from build123d import *

# Parameters (mm, degrees)
EXTRUDE_1_DEPTH = 3


with BuildPart() as part:
    # 草图1 → 凸台-拉伸1 (new body)
    with BuildSketch(Plane(origin=(0, 0, 0), x_dir=(-1, 0, 0), z_dir=(0, 0, 1))):
        with BuildLine():
            Line((-132.77617551, 2.029328632), (-134.77617551, 4.029328632))
            Line((-134.77617551, 4.029328632), (-144.77617551, 4.029328632))
            Line((-144.77617551, 4.029328632), (-144.77617551, 0.948486637))
            Line((-144.77617551, 0.948486637), (-156.77617551, 0.948486637))
            Line((-156.77617551, 0.948486637), (-156.77617551, 4.029328632))
            Line((-156.77617551, 4.029328632), (-181.77617551, 4.029328632))
            Line((-181.77617551, 4.029328632), (-181.77617551, 0.948486637))
            Line((-181.77617551, 0.948486637), (-195.77617551, 0.948486637))
            Line((-195.77617551, 0.948486637), (-195.77617551, 5.029328632))
            Line((-195.77617551, 5.029328632), (-207.77617551, 5.029328632))
            Line((-207.77617551, 5.029328632), (-207.77617551, 0.948486637))
            Line((-207.77617551, 0.948486637), (-221.77617551, 0.948486637))
            Line((-221.77617551, 0.948486637), (-221.77617551, 4.029328632))
            Line((-221.77617551, 4.029328632), (-246.77617551, 4.029328632))
            Line((-246.77617551, 4.029328632), (-246.77617551, 0.948486637))
            Line((-246.77617551, 0.948486637), (-258.77617551, 0.948486637))
            Line((-258.77617551, 0.948486637), (-258.77617551, 4.029328632))
            Line((-258.77617551, 4.029328632), (-268.77617551, 4.029328632))
            Line((-268.77617551, 4.029328632), (-270.77617551, 2.029328632))
            Line((-270.77617551, 2.029328632), (-270.77617551, -41.970671368))
            ThreePointArc((-270.77617551, -41.970671368), (-272.240641604, -45.506205274), (-275.77617551, -46.970671368))
            Line((-275.77617551, -46.970671368), (-296.77617551, -46.970671368))
            ThreePointArc((-296.77617551, -46.970671368), (-298.190389072, -47.556457806), (-298.77617551, -48.970671368))
            Line((-298.77617551, -48.970671368), (-298.77617551, -61.470671368))
            ThreePointArc((-298.77617551, -61.470671368), (-292.125960742, -70.210089556), (-282.77617551, -75.970671368))
            Line((-282.77617551, -75.970671368), (-274.77617551, -75.970671368))
            Line((-274.77617551, -75.970671368), (-272.77617551, -73.970671368))
            Line((-272.77617551, -73.970671368), (-272.77617551, -66.665321612))
            ThreePointArc((-272.77617551, -66.665321612), (-271.897495853, -64.544001269), (-269.77617551, -63.665321612))
            Line((-269.77617551, -63.665321612), (-266.77617551, -63.665321612))
            Line((-266.77617551, -63.665321612), (-266.77617551, -53.665321612))
            Line((-266.77617551, -53.665321612), (-262.77617551, -53.665321612))
            Line((-262.77617551, -53.665321612), (-262.77617551, -63.665321612))
            Line((-262.77617551, -63.665321612), (-248.77617551, -63.665321612))
            Line((-248.77617551, -63.665321612), (-242.77617551, -57.665321612))
            Line((-242.77617551, -57.665321612), (-242.77617551, -19.470671368))
            Line((-242.77617551, -19.470671368), (-235.77617551, -19.470671368))
            Line((-235.77617551, -19.470671368), (-235.77617551, -25.415321612))
            Line((-235.77617551, -25.415321612), (-231.17617551, -25.415321612))
            Line((-231.17617551, -25.415321612), (-231.17617551, -23.370671368))
            Line((-231.17617551, -23.370671368), (-232.22617551, -23.370671368))
            ThreePointArc((-232.22617551, -23.370671368), (-232.438307544, -23.282803402), (-232.52617551, -23.070671368))
            Line((-232.52617551, -23.070671368), (-232.52617551, -21.170671368))
            ThreePointArc((-232.52617551, -21.170671368), (-232.438307544, -20.958539334), (-232.22617551, -20.870671368))
            Line((-232.22617551, -20.870671368), (-231.12617551, -20.870671368))
            Line((-231.12617551, -20.870671368), (-231.12617551, -20.670671368))
            ThreePointArc((-231.12617551, -20.670671368), (-231.038307544, -20.458539334), (-230.82617551, -20.370671368))
            Line((-230.82617551, -20.370671368), (-228.72617551, -20.370671368))
            ThreePointArc((-228.72617551, -20.370671368), (-228.514043475, -20.458539334), (-228.42617551, -20.670671368))
            Line((-228.42617551, -20.670671368), (-228.42617551, -20.870671368))
            Line((-228.42617551, -20.870671368), (-227.32617551, -20.870671368))
            ThreePointArc((-227.32617551, -20.870671368), (-227.114043475, -20.958539334), (-227.02617551, -21.170671368))
            Line((-227.02617551, -21.170671368), (-227.02617551, -23.070671368))
            ThreePointArc((-227.02617551, -23.070671368), (-227.114043475, -23.282803402), (-227.32617551, -23.370671368))
            Line((-227.32617551, -23.370671368), (-228.37617551, -23.370671368))
            Line((-228.37617551, -23.370671368), (-228.37617551, -25.415321612))
            Line((-228.37617551, -25.415321612), (-224.77617551, -25.415321612))
            Line((-224.77617551, -25.415321612), (-224.77617551, -30.915321612))
            Line((-224.77617551, -30.915321612), (-214.77617551, -30.915321612))
            Line((-214.77617551, -30.915321612), (-214.77617551, -25.415321612))
            Line((-214.77617551, -25.415321612), (-203.17617551, -25.415321612))
            Line((-203.17617551, -25.415321612), (-203.17617551, -23.370671368))
            Line((-203.17617551, -23.370671368), (-204.22617551, -23.370671368))
            ThreePointArc((-204.22617551, -23.370671368), (-204.438307544, -23.282803402), (-204.52617551, -23.070671368))
            Line((-204.52617551, -23.070671368), (-204.52617551, -21.170671368))
            ThreePointArc((-204.52617551, -21.170671368), (-204.438307544, -20.958539334), (-204.22617551, -20.870671368))
            Line((-204.22617551, -20.870671368), (-203.12617551, -20.870671368))
            Line((-203.12617551, -20.870671368), (-203.12617551, -20.670671368))
            ThreePointArc((-203.12617551, -20.670671368), (-203.038307544, -20.458539334), (-202.82617551, -20.370671368))
            Line((-202.82617551, -20.370671368), (-200.72617551, -20.370671368))
            ThreePointArc((-200.72617551, -20.370671368), (-200.514043475, -20.458539334), (-200.42617551, -20.670671368))
            Line((-200.42617551, -20.670671368), (-200.42617551, -20.870671368))
            Line((-200.42617551, -20.870671368), (-199.32617551, -20.870671368))
            ThreePointArc((-199.32617551, -20.870671368), (-199.114043475, -20.958539334), (-199.02617551, -21.170671368))
            Line((-199.02617551, -21.170671368), (-199.02617551, -23.070671368))
            ThreePointArc((-199.02617551, -23.070671368), (-199.114043475, -23.282803402), (-199.32617551, -23.370671368))
            Line((-199.32617551, -23.370671368), (-200.37617551, -23.370671368))
            Line((-200.37617551, -23.370671368), (-200.37617551, -25.415321612))
            Line((-200.37617551, -25.415321612), (-188.77617551, -25.415321612))
            Line((-188.77617551, -25.415321612), (-188.77617551, -30.915321612))
            Line((-188.77617551, -30.915321612), (-178.77617551, -30.915321612))
            Line((-178.77617551, -30.915321612), (-178.77617551, -25.415321612))
            Line((-178.77617551, -25.415321612), (-175.17617551, -25.415321612))
            Line((-175.17617551, -25.415321612), (-175.17617551, -23.370671368))
            Line((-175.17617551, -23.370671368), (-176.22617551, -23.370671368))
            ThreePointArc((-176.22617551, -23.370671368), (-176.438307544, -23.282803402), (-176.52617551, -23.070671368))
            Line((-176.52617551, -23.070671368), (-176.52617551, -21.170671368))
            ThreePointArc((-176.52617551, -21.170671368), (-176.438307544, -20.958539334), (-176.22617551, -20.870671368))
            Line((-176.22617551, -20.870671368), (-175.12617551, -20.870671368))
            Line((-175.12617551, -20.870671368), (-175.12617551, -20.670671368))
            ThreePointArc((-175.12617551, -20.670671368), (-175.038307544, -20.458539334), (-174.82617551, -20.370671368))
            Line((-174.82617551, -20.370671368), (-172.72617551, -20.370671368))
            ThreePointArc((-172.72617551, -20.370671368), (-172.514043475, -20.458539334), (-172.42617551, -20.670671368))
            Line((-172.42617551, -20.670671368), (-172.42617551, -20.870671368))
            Line((-172.42617551, -20.870671368), (-171.32617551, -20.870671368))
            ThreePointArc((-171.32617551, -20.870671368), (-171.114043475, -20.958539334), (-171.02617551, -21.170671368))
            Line((-171.02617551, -21.170671368), (-171.02617551, -23.070671368))
            ThreePointArc((-171.02617551, -23.070671368), (-171.114043475, -23.282803402), (-171.32617551, -23.370671368))
            Line((-171.32617551, -23.370671368), (-172.37617551, -23.370671368))
            Line((-172.37617551, -23.370671368), (-172.37617551, -25.415321612))
            Line((-172.37617551, -25.415321612), (-167.77617551, -25.415321612))
            Line((-167.77617551, -25.415321612), (-167.77617551, -19.470671368))
            Line((-167.77617551, -19.470671368), (-160.77617551, -19.470671368))
            Line((-160.77617551, -19.470671368), (-160.77617551, -57.665321612))
            Line((-160.77617551, -57.665321612), (-154.77617551, -63.665321612))
            Line((-154.77617551, -63.665321612), (-140.77617551, -63.665321612))
            Line((-140.77617551, -63.665321612), (-140.77617551, -53.665321612))
            Line((-140.77617551, -53.665321612), (-136.77617551, -53.665321612))
            Line((-136.77617551, -53.665321612), (-136.77617551, -63.665321612))
            Line((-136.77617551, -63.665321612), (-133.77617551, -63.665321612))
            ThreePointArc((-133.77617551, -63.665321612), (-131.654855166, -64.544001269), (-130.77617551, -66.665321612))
            Line((-130.77617551, -66.665321612), (-130.77617551, -73.970671368))
            Line((-130.77617551, -73.970671368), (-128.77617551, -75.970671368))
            Line((-128.77617551, -75.970671368), (-120.77617551, -75.970671368))
            ThreePointArc((-120.77617551, -75.970671368), (-111.426390277, -70.210089556), (-104.77617551, -61.470671368))
            Line((-104.77617551, -61.470671368), (-104.77617551, -48.970671368))
            ThreePointArc((-104.77617551, -48.970671368), (-105.361961947, -47.556457806), (-106.77617551, -46.970671368))
            Line((-106.77617551, -46.970671368), (-127.77617551, -46.970671368))
            ThreePointArc((-127.77617551, -46.970671368), (-131.311709416, -45.506205274), (-132.77617551, -41.970671368))
            Line((-132.77617551, -41.970671368), (-132.77617551, 2.029328632))
        make_face()
        with BuildLine():
            Line((-187.141847312, -9.202827725), (-181.907913386, -11.645330223))
            ThreePointArc((-181.907913386, -11.645330223), (-181.354534763, -12.768096904), (-182.330798852, -13.551513363))
            Line((-182.330798852, -13.551513363), (-188.27617551, -13.551513363))
            ThreePointArc((-188.27617551, -13.551513363), (-188.983282291, -13.258620144), (-189.27617551, -12.551513363))
            Line((-189.27617551, -12.551513363), (-189.27617551, -10.562102435))
            ThreePointArc((-189.27617551, -10.562102435), (-188.58193841, -9.296896464), (-187.141847312, -9.202827725))
        make_face(mode=Mode.SUBTRACT)
        with BuildLine():
            Line((-221.644437633, -11.645330223), (-216.410503708, -9.202827725))
            ThreePointArc((-216.410503708, -9.202827725), (-214.970412609, -9.296896464), (-214.27617551, -10.562102435))
            Line((-214.27617551, -10.562102435), (-214.27617551, -12.551513363))
            ThreePointArc((-214.27617551, -12.551513363), (-214.569068729, -13.258620144), (-215.27617551, -13.551513363))
            Line((-215.27617551, -13.551513363), (-221.221552168, -13.551513363))
            ThreePointArc((-221.221552168, -13.551513363), (-222.197816256, -12.768096904), (-221.644437633, -11.645330223))
        make_face(mode=Mode.SUBTRACT)
    extrude(amount=EXTRUDE_1_DEPTH)


solid = part.part
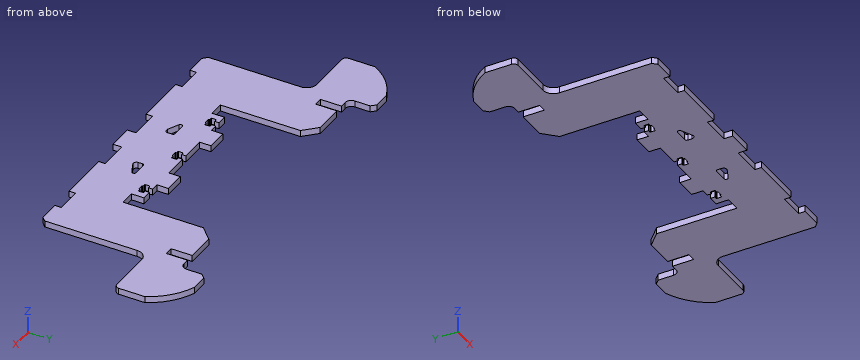
Read the model definition and answer for the solid it produces. Units are mm, in the model's axes. Round coordinates to 2 decimals unless told otherwise and drop trailing zeros. Write each loop counter-clockwise with the first axis right and the second up, starting at its lowest first coordinate (ties: lowest second). Pieces come first, ordered by that corner, then holes. Notation, with made-up numbers: (72, 20) - (82, 20) arc R24 ccw to (82, 44) - close; hole circle Ø7 at (-10, 29.25). An arc over 180 degrees is marked (long way). One line per question, with ' | ' between items. Start each with the question number.
1. Section D-D (x = 261) is taken. Determine the outline of the cut face in (y, z), and give its area (3 significant figures).
2. Section C-C (y = 70) is taken. Determine the outline of the cut face in (x, z).
3. Section A-A (y = 36) is taken. Determine the outline of the cut face in (x, z), and give its area (3 significant figures).
4. Find the intervals of material crossed by probe 1 along X at (y, z) = (-1, 0.8); probe 2 along X at (y, z) = (23, 2.8); probe 3 along X at (y, z) = (54.5, 1.65), in increasing order. Write a range as [from, to].
5. Each of these flat-tipped pins is pushed along its axis until it touches: pin 1 (1.5 mm diameter, centred on y = 19.5, z = 1.5, fed in from -X); pin 2 (0.6 mm diameter, centred on y = 22, z = 2, fed in from +X); pin 3 (1.5 mm diameter, centred on x = 183.5, z = 2, fed in from +Y). Where does it stop, or does it pass through?
6. Section B-B (z = 1.85) is taken. Give the number of separate pieces and of enclosed holes in the cut face, and give its area (3 significant figures).
Filled in:
1) outline: (-4.03, 0) - (63.67, 0) - (63.67, 3) - (-4.03, 3) - close | area: 203 mm²
2) outline: (111.2, 0) - (130.78, 0) - (130.78, 3) - (111.2, 3) - close; (272.78, 0) - (292.36, 0) - (292.36, 3) - (272.78, 3) - close
3) outline: (132.78, 0) - (160.78, 0) - (160.78, 3) - (132.78, 3) - close; (242.78, 0) - (270.78, 0) - (270.78, 3) - (242.78, 3) - close | area: 168 mm²
4) probe 1: [132.78, 144.78], [156.78, 181.78], [195.78, 207.78], [221.78, 246.78], [258.78, 270.78] | probe 2: [132.78, 160.78], [167.78, 171.03], [176.53, 199.03], [204.53, 227.03], [232.53, 235.78], [242.78, 270.78] | probe 3: [104.78, 136.78], [140.78, 160.78], [242.78, 262.78], [266.78, 298.78]
5) pin 1: x = 132.78 | pin 2: x = 270.78 | pin 3: y = 30.92
6) separate pieces: 1 | enclosed holes: 2 | area: 7,260 mm²
